```python
from build123d import *

# Parameters (mm, degrees)
SKETCH1_W            = 103.968410754
SKETCH1_H            = 34.186058554
BOSS_EXTRUDE1_DEPTH  = 15
SKETCH2_W            = 103.968410754
SKETCH2_H            = 14.786910166
BOSS_EXTRUDE2_DEPTH  = 60
CUT_EXTRUDE1_DEPTH   = 94.826164315
M4_CLEARANCE_HOLE1_D = 4.5
M4_CLEARANCE_HOLE2_D = 4.5


with BuildPart() as part:
    # Sketch1 → Boss-Extrude1 (new body)
    with BuildSketch(Plane.XY):
        with Locations((-17.492568813, 2.403154481)):
            Rectangle(SKETCH1_W, SKETCH1_H)
    extrude(amount=BOSS_EXTRUDE1_DEPTH)

    # Sketch2 → Boss-Extrude2 (add)
    with BuildSketch(Plane(origin=(0, 0, 0), x_dir=(-1, 0, 0), z_dir=(0, 0, -1))):
        with Locations((17.492568813, 12.102728675)):
            Rectangle(SKETCH2_W, SKETCH2_H)
    extrude(amount=BOSS_EXTRUDE2_DEPTH)

    # Sketch3 → Cut-Extrude1 (cut, through all)
    with BuildSketch(Plane.XZ.offset(-4.709273592)):
        Polygon((-45.441256031, 0), (-45.441256031, -15.4), (-4.909163254, -53.722384085), (17.34490568, -53.722384085), (17.34490568, 0), (34.491636564, 0), (34.491636564, -60), (-69.47677419, -60), (-69.47677419, 0), align=None)
    extrude(amount=-CUT_EXTRUDE1_DEPTH, mode=Mode.SUBTRACT)

    # M4 Clearance Hole1 (through all)
    with Locations(Plane(origin=(-9.237078097, 4.709273592, -22.640821114), x_dir=(-1, 0, 0), z_dir=(0, -1, 0))):
        with Locations((0, 0), (15.604992815, -15.604992814)):
            Hole(M4_CLEARANCE_HOLE1_D / 2)

    # M4 Clearance Hole2 (through all)
    with Locations(Plane(origin=(-57.782319431, 1.498461161, 0), x_dir=(-1, 0, 0), z_dir=(0, 0, -1))):
        with Locations((0, 0), (-78.208808727, 0)):
            Hole(M4_CLEARANCE_HOLE2_D / 2)


solid = part.part
```
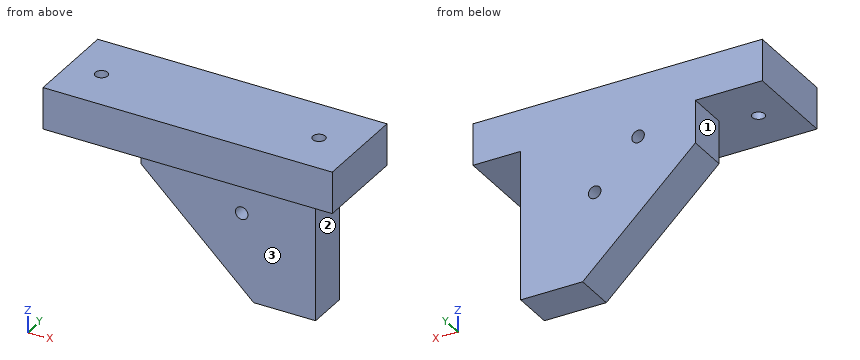
Source: CAD feature listing. Evaluate the final solid. Frame: model axes, mm. Face numbers are marked on the shaded views. A direction names the side the tool comes from. Give positions to 0.01 mm unless a question says otherwise; leave off trailing zeros. Loops run counter-clockwise (first coordinate to the right, second up) from the corner with the lowest first, then second, coordinate; pieces in that order, holes last. Notation, with made-up numbers: (6, 59) - (61, 59) arc R15 cw to (61, 71) - close; hole circle Ø4 at (70, 50.25). An arc over 180 degrees is marked (long way). Use CSV: the item, a comma, the result in double quotes.
1) Cut plane B-B (y = 6.5). Output: boundary loops of the cut face in (x, z).
Worked out:
outline,"(-69.48, 0) - (-45.44, 0) - (-45.44, -15.4) - (-4.91, -53.72) - (17.34, -53.72) - (17.34, 0) - (34.49, 0) - (34.49, 15) - (-69.48, 15) - close; hole circle Ø4.5 at (-24.84, -7.04); hole circle Ø4.5 at (-9.24, -22.64)"
2) Pin query (flat end, axial travel): P1, Ø1, axis at x = -14.5, z = -1.5, coming from the -Y side; P2, Ø2, axis at x = -2.5, y = -8.5, coming from the -Z side; P3, Ø4.5, axis at y = 9.5, z = -7, coming from the -X side; P4, Ø2.5, axis at x = -24.84, z = -7.04, coming from the +Y side. Return the tip coordinate at first contact, or that it passes through.
Worked out:
P1,"stops at y = 4.71"
P2,"stops at z = 0"
P3,"stops at x = -45.44"
P4,"passes through"
3) Line query: line 1 (X direction, y = 11, z = -11); line 2 (Y direction, x = -20, z = -39); line 3 (Z direction, x = -25, y = 14). Output: solid intervals per line, ascending.
Worked out:
line 1,"x = -45.44 to 17.34"
line 2,"y = 4.71 to 19.5"
line 3,"z = -34.73 to -9.28, -4.79 to 15"
4) Cut plane A-A (x = 8). Output: boundary loops of the cut face in (y, z).
Worked out:
outline,"(-14.69, 0) - (4.71, 0) - (4.71, -53.72) - (19.5, -53.72) - (19.5, 15) - (-14.69, 15) - close"
5) Set-up query: the marked faces 1, 2 and 3. Return all of +Z, -Z, +X, -X, +Y, -Y with unobstructed straight access to the full face (end or side cutting, diameter ignored); none if empty.
Worked out:
face 1,"-Z, -X, +Y, -Y"
face 2,"-Z, +X, +Y, -Y"
face 3,"-Z, +X, -X, -Y"
6) Cut plane C-C (y = -10). Output: boundary loops of the cut face in (x, z).
Worked out:
outline,"(-69.48, 0) - (34.49, 0) - (34.49, 15) - (-69.48, 15) - close"
7) Cut plane D-D (z = -14). Output: boundary loops of the cut face in (x, y).
Worked out:
outline,"(-45.44, 4.71) - (17.34, 4.71) - (17.34, 19.5) - (-45.44, 19.5) - close"
